The model under review builds one solid part; all positions refer to its coordinate system, in mm. Face numbers are marked on the shaded views. A direction names the side the tool comes from. Give positions to 0.01 mm unless a question says otherwise; leave off trailing zeros. Write each loop counter-clockwise with the first axis right and the second up, starting at its lowest first coordinate (ties: lowest second). Pieces come first, ordered by that corner, then holes. Notation, with made-up numbers: (82, -21.5) -> (112, -21.5) arc R27 ccw to (112, -0.5) -> close; hole circle Ø9 at (55.5, -11.5). An arc over 180 degrees is marked (long way). Use CSV: the item, a comma, the result in double quotes.
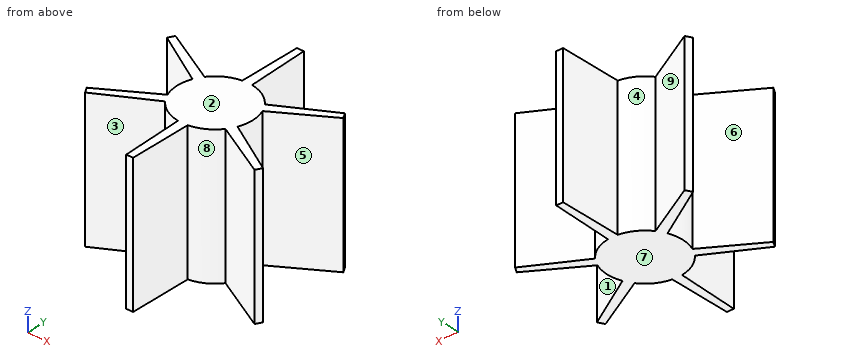
```python
from build123d import *

# Parameters (mm, degrees)
BOSS_EXTRUDE1_DEPTH = 100


with BuildPart() as part:
    # Sketch1 → Boss-Extrude1 (new body)
    with BuildSketch(Plane.XY):
        with BuildLine():
            Line((3.5, 27.12898754), (2.5, 72))
            Line((2.5, 72), (-2.5, 72))
            Line((-2.5, 72), (-3.5, 27.12898754))
            ThreePointArc((-3.5, 27.12898754), (-13.676914536, 23.689110868), (-21.744392388, 16.595582683))
            Line((-21.744392388, 16.595582683), (-61.103829072, 38.165063509))
            Line((-61.103829072, 38.165063509), (-63.603829072, 33.834936491))
            Line((-63.603829072, 33.834936491), (-25.244392388, 10.533404857))
            ThreePointArc((-25.244392388, 10.533404857), (-27.353829072, 0), (-25.244392388, -10.533404857))
            Line((-25.244392388, -10.533404857), (-63.603829072, -33.834936491))
            Line((-63.603829072, -33.834936491), (-61.103829072, -38.165063509))
            Line((-61.103829072, -38.165063509), (-21.744392388, -16.595582683))
            ThreePointArc((-21.744392388, -16.595582683), (-13.676914536, -23.689110868), (-3.5, -27.12898754))
            Line((-3.5, -27.12898754), (-2.5, -72))
            Line((-2.5, -72), (2.5, -72))
            Line((2.5, -72), (3.5, -27.12898754))
            ThreePointArc((3.5, -27.12898754), (13.676914536, -23.689110868), (21.744392388, -16.595582683))
            Line((21.744392388, -16.595582683), (61.103829072, -38.165063509))
            Line((61.103829072, -38.165063509), (63.603829072, -33.834936491))
            Line((63.603829072, -33.834936491), (25.244392388, -10.533404857))
            ThreePointArc((25.244392388, -10.533404857), (27.353829072, 0), (25.244392388, 10.533404857))
            Line((25.244392388, 10.533404857), (63.603829072, 33.834936491))
            Line((63.603829072, 33.834936491), (61.103829072, 38.165063509))
            Line((61.103829072, 38.165063509), (21.744392388, 16.595582683))
            ThreePointArc((21.744392388, 16.595582683), (13.676914536, 23.689110868), (3.5, 27.12898754))
        make_face()
    extrude(amount=BOSS_EXTRUDE1_DEPTH)


solid = part.part
```
Q1. To check wall thickness, follow probe 1 along X at (y, z) = (35.5, 57); probe 2 along X at (y, z) = (24.5, 95.5); probe 3 along Y at (x, z) = (-29.5, 68.5). State the ranges of each line that lie inside material, in increasing order.
Derived:
probe 1,"x = -62.64 to -56.24, -3.31 to 3.31, 56.24 to 62.64"
probe 2,"x = -48.24 to -36.17, -12.16 to 12.16, 36.17 to 48.24"
probe 3,"y = -20.85 to -13.12, 13.12 to 20.85"
Q2. Consider section A-A (z = 77). Write out the cut boundary in (x, y), then the cut area to 3 significant figures.
Derived:
outline,"(-63.6, -33.83) -> (-61.1, -38.17) -> (-21.74, -16.6) arc R27.35 ccw to (-3.5, -27.13) -> (-2.5, -72) -> (2.5, -72) -> (3.5, -27.13) arc R27.35 ccw to (21.74, -16.6) -> (61.1, -38.17) -> (63.6, -33.83) -> (25.24, -10.53) arc R27.35 ccw to (25.24, 10.53) -> (63.6, 33.83) -> (61.1, 38.17) -> (21.74, 16.6) arc R27.35 ccw to (3.5, 27.13) -> (2.5, 72) -> (-2.5, 72) -> (-3.5, 27.13) arc R27.35 ccw to (-21.74, 16.6) -> (-61.1, 38.17) -> (-63.6, 33.83) -> (-25.24, 10.53) arc R27.35 ccw to (-25.24, -10.53) -> close"
area,"3,960 mm2"
Q3. The part is to be moulded in two halves that separate along X. For the marked faces 1, 2, 3 and 4, say which applies: pulls with the +X half, pulls with the -X half, needs draft (parallel to the pull), parting line crosses it, or undercut.
Derived:
face 1,"pulls with the +X half"
face 2,"needs draft"
face 3,"undercut"
face 4,"undercut"
Q4. Consider section B-B (x = 40). Write out the cut boundary in (y, z), then the cut area to 3 significant figures.
Derived:
outline,"(-26.6, 0) -> (-19.5, 0) -> (-19.5, 100) -> (-26.6, 100) -> close; (19.5, 0) -> (26.6, 0) -> (26.6, 100) -> (19.5, 100) -> close"
area,"1,420 mm2"
Q5. Insertion check: pin 1 (12 mm diameter, centred on y = -56.5, z = 35.5, fed in from -X); pin 2 (3 mm diameter, centred on y = -44.5, z = 77, fed in from +X); pin 3 (1.5 mm diameter, centred on x = 47, z = 39, fed in from -Y). Each pin has a flat end and moves straight along its axis. Give the tip position at first contact, or say it passes through.
Derived:
pin 1,"stops at x = -2.98"
pin 2,"stops at x = 3.15"
pin 3,"stops at y = -30.85"
Q6. Consider section D-D (x = -31). Write out the cut boundary in (y, z), then the cut area to 3 significant figures.
Derived:
outline,"(-21.67, 0) -> (-14.03, 0) -> (-14.03, 100) -> (-21.67, 100) -> close; (14.03, 0) -> (21.67, 0) -> (21.67, 100) -> (14.03, 100) -> close"
area,"1,530 mm2"
Q7. Machinability: for the marked faces 5, 6, 7, 8 and 9, which of the approach directions +Z, -Z, +X, -X, +Y, -Y give a long, thin tool a straight path to every point of the face, cutting with its end or side? Answer none if there is none.
Derived:
face 5,"+Z, -Z, +X"
face 6,"+Z, -Z, -X"
face 7,"-Z, +X, -X, +Y, -Y"
face 8,"+Z, -Z, -Y"
face 9,"+Z, -Z, +Y"
Q8. Consider section C-C (y = -21.5). Write out the cut boundary in (x, z).
Derived:
outline,"(-43.3, 0) -> (-30.69, 0) -> (-30.69, 100) -> (-43.3, 100) -> close; (-16.91, 0) -> (16.91, 0) -> (16.91, 100) -> (-16.91, 100) -> close; (30.69, 0) -> (43.3, 0) -> (43.3, 100) -> (30.69, 100) -> close"
